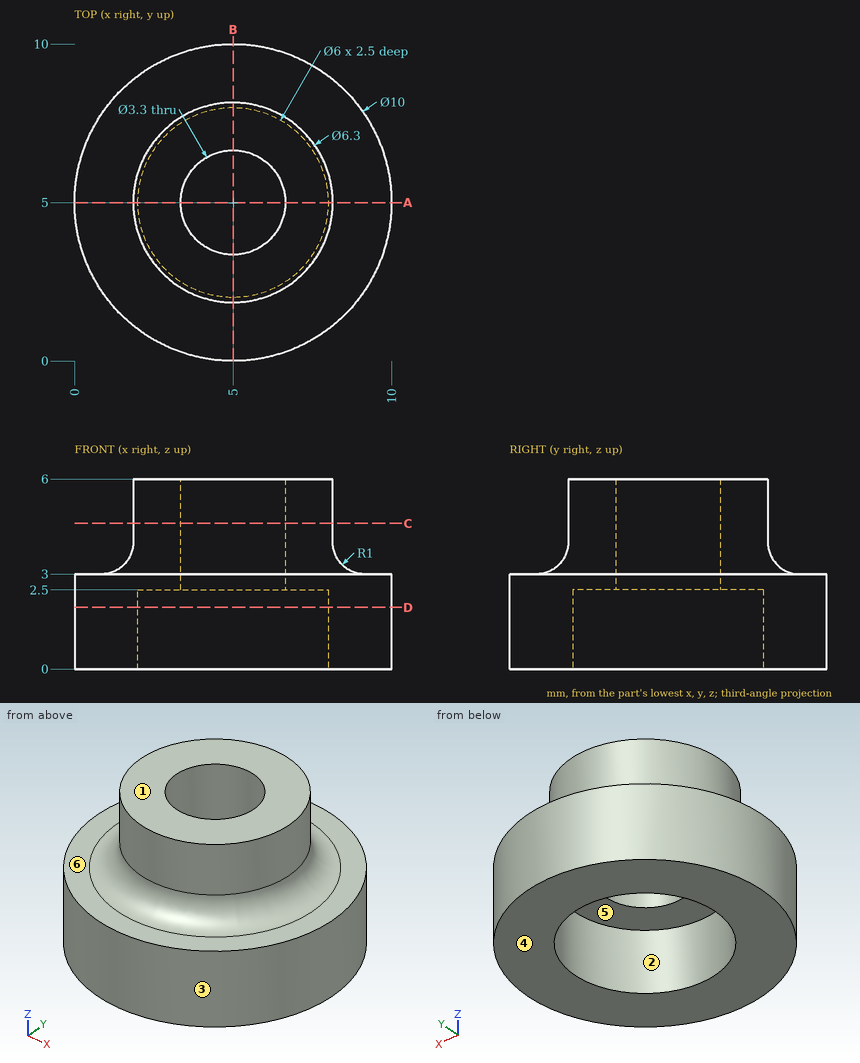
Job drawing, mm, ordinate dimensions from the low corner. One solid piece. A direction names the side the tool comes from. Round coordinates to 2 decimals unless told otherwise and drop trailing zeros. Loops run counter-clockwise (first coordinate to the right, second up) from the corner with the lowest first, then second, coordinate; pieces in that order, holes last. Notation, with made-up numbers: (-1.75, 82.5) -> (14.25, 82.5) arc R21 ccw to (14.25, 113.5) -> close; hole circle Ø10 at (-23, 70.5). An arc over 180 degrees is marked (long way). Use CSV: the item, a comma, the result in double quotes. Start each with the question number.
Q1. Saw through at C-C on z = 4.6. Give the cut face in (x, y), and give its area (3 significant figures).
Q2. Which spindle directions (+Z, -Z, +X, -X, +Y, -Y) get a long thin tool onto all of the face, cutting with end or side? Do the marked faces 4, 5 and 6. Say none if no direction does.
Q3. Saw through at A-A on y = 5. Give the cut face in (x, z).
Q4. Mould opens along X. For the marked faces 1, 2 and 3 say: +X half, -X half, draft (parallel to the pull), parting line (faces both ways), or undercut.
Q5. Drill centre lines: L1, parallel to Y at x = 5, z = 5.1; L2, parallel to Y at x = 1, z = 2.45; L3, parallel to Z at x = 1, y = 6. Where is each one in solid material? Low to high.
Q6. Saw through at D-D on z = 1.95. Give the cut face in (x, y).
Q7. Flat gauge pins, fed straight in: pin 1 Ø1.5 at (x, z) = (8, 3) entering from -Y; pin 2 Ø2 at (y, z) = (2.5, 3) entering from +X; pin 3 Ø3 at (x, y) = (5, 5) entering from -Z (1 decimal); pin 4 Ø1.5 at (x, z) = (3.5, 3) entering from +Y. Where does each tip first touch, or does it go through?
Solutions:
1,outline,"circle Ø6.3 at (5, 5); hole circle Ø3.3 at (5, 5)"
1,area,"22.6 mm^2"
2,face 4,"-Z, +X, -X, +Y, -Y"
2,face 5,"-Z"
2,face 6,"+Z"
3,outline,"(0, 0) -> (2, 0) -> (2, 2.5) -> (3.35, 2.5) -> (3.35, 6) -> (1.85, 6) -> (1.85, 4) arc R1 cw to (0.85, 3) -> (0, 3) -> close; (6.65, 2.5) -> (8, 2.5) -> (8, 0) -> (10, 0) -> (10, 3) -> (9.15, 3) arc R1 cw to (8.15, 4) -> (8.15, 6) -> (6.65, 6) -> close"
4,face 1,"draft"
4,face 2,"undercut"
4,face 3,"parting line"
5,L1,"y = 1.85 to 3.35, 6.65 to 8.15"
5,L2,"y = 2 to 8"
5,L3,"z = 0 to 3"
6,outline,"circle Ø10 at (5, 5); hole circle Ø6 at (5, 5)"
7,pin 1,"stops at y = 0.53"
7,pin 2,"stops at x = 9.77"
7,pin 3,"passes through"
7,pin 4,"stops at y = 9.94"
